Autodesk Fusion 360 part; units mm, degrees
sketch "Esquisse1" plane through (0, 0, 0) normal (0, 0, 1) x (1, 0, 0)
  circle A0 centre (0, 0) radius 1.75
  circle A1 centre (0, 0) radius 4
  circle A2 centre (0, 0) radius 7
  dimension "d1" = 3.5
  dimension "d10" = 8
  dimension "d11" = 3
extrude "Extrusion2" add sketch "Esquisse1" along normal blind 5 contours A1
extrude "Extrusion3" add sketch "Esquisse1" along normal blind 2 contours A2
mirror "Symétrie miroir2" about plane through (0, 0, 5) normal (0, 0, 1) of bodies 1 merged
Can you work these out from the model? Positions are in its coordinate system, mm. A direction names the side the tool comes from. Coordinates: 2 decimals unless noted, no trailing zeros. Loops run counter-clockwise (first coordinate to the right, second up) from the corner with the lowest first, then second, coordinate; pieces in that order, holes last.
1) Imagine slicing it at C-C on z = 3. List the corners of the cut face in (x, y) for me, plus the area to 3 significant figures.
2) Imagine slicing it at D-D on y = 4.75. List the corners of the cut face in (x, z) for me.
3) Thinking about a two-plate mould opening in Z: for faces 3 (the flat face through (1.5, -1.5, 0)), 4 (the cylindrical face through (6.466, -2.681, 9.014)), 5 (the flat face through (3, -3, 2)), 6 (the flat face through (-1.5, -1.5, 10)), which applies, pulls with the +Z half, pulls with the -Z half, needs draft (parallel to the pull), parting line crosses it, or undercut?
4) I need wall thicknesses on probe 1 along Z at (x, y) = (-4, 5); probe 2 along Y at (x, z) = (0, 6); probe 3 along X at (y, z) = (-1, 6.75). Which ranges of each line are inside material? Lowest first, please.
5) Which directions (+Z, -Z, +X, -X, +Y, -Y) give clear straight access to the entire face, cutting with the end or side of a thin tool? Please do faces 1 (the cylindrical face through (-0.867, -3.905, 5.042)), 2 (the cylindrical face through (1.617, -0.67, 5.07)).
6) For pin 1 (5 mm diameter, centred on x = -4.5, z = 5, fed in from +Y); pin 2 (1.5 mm diameter, centred on y = 1, z = 4.5, fed in from +X); pin 3 (3 mm diameter, centred on x = -2.5, z = 4.5, fed in from +Y), each with a flat end and sliding along its axis, tell me the tip position at first contact or that it passes through.
7) Imagine slicing it at A-A on y = 0. List the corners of the cut face in (x, z) for me.
Completed:
1. outline: circle Ø8 at (0, 0); hole circle Ø3.5 at (0, 0)
1. area: 40.6 mm2
2. outline: (-5.14, 0) - (5.14, 0) - (5.14, 2) - (-5.14, 2) - close; (-5.14, 8) - (5.14, 8) - (5.14, 10) - (-5.14, 10) - close
3. face 3: pulls with the -Z half
3. face 4: needs draft
3. face 5: undercut
3. face 6: pulls with the +Z half
4. probe 1: z = 0 to 2, 8 to 10
4. probe 2: y = -4 to -1.75, 1.75 to 4
4. probe 3: x = -3.87 to -1.44, 1.44 to 3.87
5. face 1: none
5. face 2: +Z, -Z
6. pin 1: stops at y = 3.46
6. pin 2: stops at x = 3.99
6. pin 3: stops at y = 3.87
7. outline: (-7, 0) - (-1.75, 0) - (-1.75, 10) - (-7, 10) - (-7, 8) - (-4, 8) - (-4, 2) - (-7, 2) - close; (1.75, 0) - (7, 0) - (7, 2) - (4, 2) - (4, 8) - (7, 8) - (7, 10) - (1.75, 10) - close
